The figure shows three views and two pictorial views of one solid part (mm, origin at its lowest corner). Answer the questions. Give positions to 0.01 mm unless a question says otherwise; leave off trailing zeros. Write each loop counter-clockwise with the first axis right and the second up, starting at its lowest first coordinate (ties: lowest second). Pieces come first, ordered by that corner, then holes. Notation, with made-up numbers: (18.25, 12.25) - (26.25, 12.25) arc R17 cw to (26.25, 29.25) - close; hole circle Ø11 at (86, -34). An arc over 180 degrees is marked (long way). Use CSV: the item, a comma, the result in double quotes. Start each with the question number.
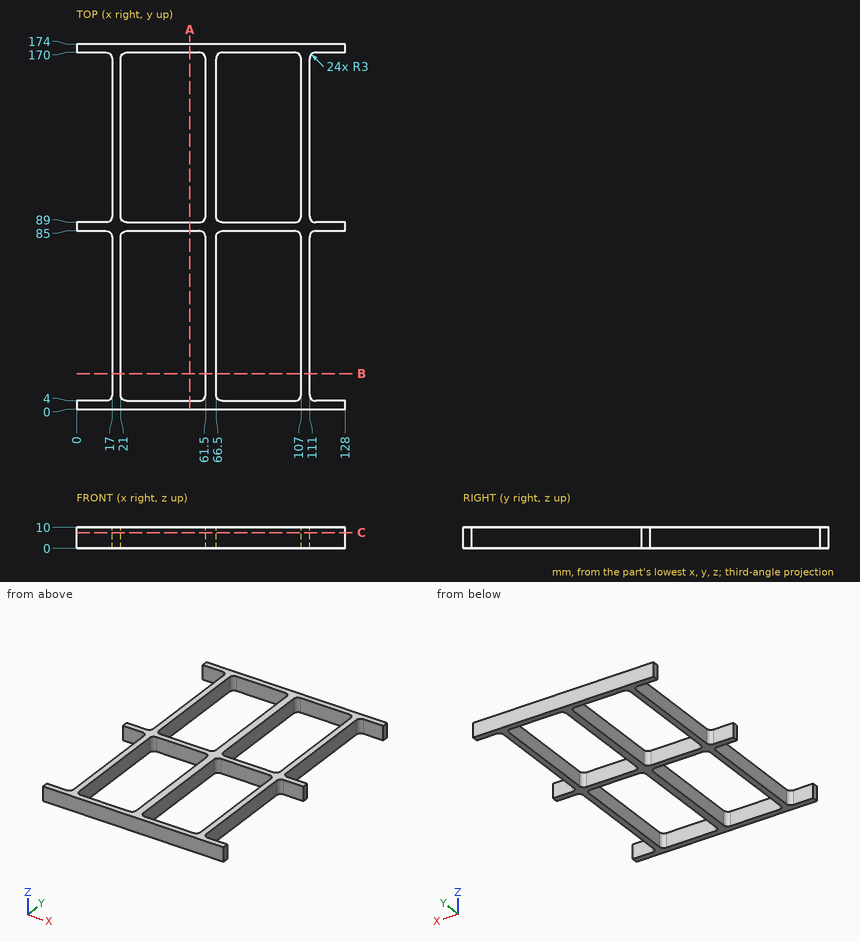
(1) Given P1, Ø5, axis at y = 142.5, z = 5.5, coming from the -X side; P2, Ø5, axis at y = 36, z = 4.5, coming from the +X side, each flat-ended and moving along its own axis, determine where each tip first touches the part or whether it passes through.
(2) Consider probe 1 along X at (y, z) = (32.5, 4.25); probe 2 along Y at (x, z) = (94, 7); probe 3 along X at (y, z) = (90.5, 3.75). Determine where each line is inside the solid, lowest interval first.
(3) The part is cut by section A-A on x = 54. Write down the section's boundary in (y, z).
(4) The part is cut by section B-B on y = 17. Write down the section's boundary in (x, z).
(5) The part is cut by section C-C on z = 7.5. Give the number of separate pieces and of enclosed holes in the cut face, plus the area to 3 significant figures.
Reported:
1,P1,"x = 17"
1,P2,"x = 111"
2,probe 1,"17 to 21, 61.5 to 66.5, 107 to 111"
2,probe 2,"0 to 4, 85 to 89, 170 to 174"
2,probe 3,"16.6 to 21.4, 61.1 to 66.9, 106.6 to 111.4"
3,outline,"(0, 0) - (4, 0) - (4, 10) - (0, 10) - close; (85, 0) - (89, 0) - (89, 10) - (85, 10) - close; (170, 0) - (174, 0) - (174, 10) - (170, 10) - close"
4,outline,"(17, 0) - (21, 0) - (21, 10) - (17, 10) - close; (61.5, 0) - (66.5, 0) - (66.5, 10) - (61.5, 10) - close; (107, 0) - (111, 0) - (111, 10) - (107, 10) - close"
5,separate pieces,"1"
5,enclosed holes,"4"
5,area,"3,690 mm²"
